For this review, take the finished solid that the model builds, in its own axes (mm). Face numbers are marked on the shaded views. Coordinates: 2 decimals unless noted, no trailing zeros. Loops run counter-clockwise (first coordinate to the right, second up) from the corner with the lowest first, then second, coordinate; pieces in that order, holes last. Notation, with made-up numbers: (86.5, 67.5) -> (112.5, 67.5) arc R10 cw to (112.5, 79.5) -> close; hole circle Ø5 at (1.5, 14). An arc over 180 degrees is marked (long way). One line per item, written item: value.
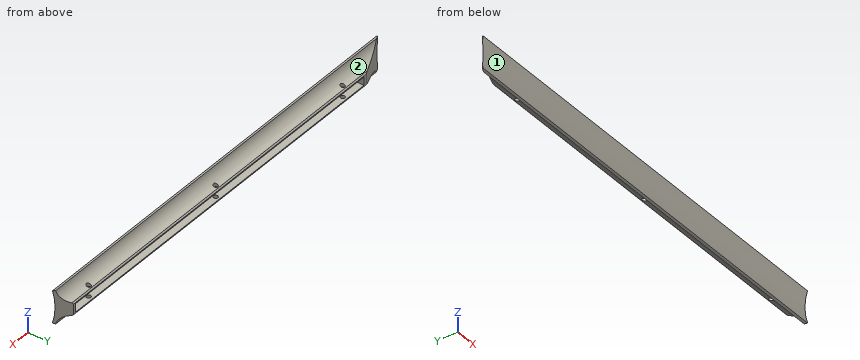
from build123d import *

# Parameters (mm, degrees)
BOSS_EXTRUDE1_DEPTH                 = 254
CUT_EXTRUDE1_DEPTH                  = 263.150751027
SKETCH3_W                           = 425.45
SKETCH3_H                           = 9.525
CUT_EXTRUDE2_DEPTH                  = 9.525
CUT_EXTRUDE3_REACH                  = 257.394
CUT_EXTRUDE3_END_RADIUS             = 15.089603758
SKETCH6_R                           = 2.4384
CUT_EXTRUDE3_DIRECTION_2_REACH      = 257.394
CUT_EXTRUDE3_DIRECTION_2_END_RADIUS = 15.089603758
CHAMFER1_SIZE                       = 1.27


with BuildPart() as part:
    # Sketch1 → Boss-Extrude1 (new, symmetric)
    with BuildSketch(Plane(origin=(0, 0, 0), x_dir=(0, 0, -1), z_dir=(1, 0, 0))):
        with BuildLine():
            Line((-7.1374, 12.7), (7.1374, 12.7))
            ThreePointArc((7.1374, 12.7), (10.363087786, 3.375642683), (18.661047774, -1.962199681))
            Line((18.661047774, -1.962199681), (18.00748716, -4.649455573))
            ThreePointArc((18.00748716, -4.649455573), (0, -2.491135768), (-18.00748716, -4.649455573))
            Line((-18.00748716, -4.649455573), (-18.661047774, -1.962199681))
            ThreePointArc((-18.661047774, -1.962199681), (-10.363087786, 3.375642683), (-7.1374, 12.7))
        make_face()
    extrude(amount=BOSS_EXTRUDE1_DEPTH, both=True)

    # Sketch2 → Cut-Extrude1 (cut, through all)
    with BuildSketch(Plane.XY.offset(44.944976028)):
        Polygon((-254, 12.7), (-215.9, 12.7), (-254, -3.6322), align=None)
        Polygon((254, -4.649455573), (224.3582, -4.649455573), (215.9, 12.7), (254, 12.7), align=None)
    extrude(amount=-CUT_EXTRUDE1_DEPTH, mode=Mode.SUBTRACT)

    # Sketch3 → Cut-Extrude2 (cut)
    with BuildSketch(Plane(origin=(0, 12.7, 0), x_dir=(1, 0, 0), z_dir=(0, 1, 0))):
        Rectangle(SKETCH3_W, SKETCH3_H)
    extrude(amount=-CUT_EXTRUDE2_DEPTH, mode=Mode.SUBTRACT)

    # Cut-Extrude3: up to this cylinder (the profile starts outside it)
    cut_extrude3_end = Plane(origin=(0, 12.7, -22.227003758), z_dir=(-1, 0, 0)) * Cylinder(CUT_EXTRUDE3_END_RADIUS, 920.617207515, mode=Mode.PRIVATE)
    # Sketch6 → Cut-Extrude3 (cut, up to the surface)
    with BuildSketch(Plane.XY.offset(-4.7625), mode=Mode.PRIVATE) as cut_extrude3_sk1:
        with Locations((-187.325, 7.9375)):
            Circle(SKETCH6_R)
    cut_extrude3_tool1 = extrude(cut_extrude3_sk1.sketch, amount=-CUT_EXTRUDE3_REACH, mode=Mode.PRIVATE) - cut_extrude3_end
    add(cut_extrude3_tool1.solids().sort_by_distance((-187.325, 7.9375, -4.7625))[0], mode=Mode.SUBTRACT)
    # Sketch6 → Cut-Extrude3 (cut, up to the surface)
    with BuildSketch(Plane.XY.offset(-4.7625), mode=Mode.PRIVATE) as cut_extrude3_sk2:
        with Locations((187.325, 7.9375)):
            Circle(SKETCH6_R)
    cut_extrude3_tool2 = extrude(cut_extrude3_sk2.sketch, amount=-CUT_EXTRUDE3_REACH, mode=Mode.PRIVATE) - cut_extrude3_end
    add(cut_extrude3_tool2.solids().sort_by_distance((187.325, 7.9375, -4.7625))[0], mode=Mode.SUBTRACT)
    # Sketch6 → Cut-Extrude3 (cut, up to the surface)
    with BuildSketch(Plane.XY.offset(-4.7625), mode=Mode.PRIVATE) as cut_extrude3_sk3:
        with Locations((0, 7.9375)):
            Circle(SKETCH6_R)
    cut_extrude3_tool3 = extrude(cut_extrude3_sk3.sketch, amount=-CUT_EXTRUDE3_REACH, mode=Mode.PRIVATE) - cut_extrude3_end
    add(cut_extrude3_tool3.solids().sort_by_distance((0, 7.9375, -4.7625))[0], mode=Mode.SUBTRACT)

    # Cut-Extrude3 direction 2: up to this cylinder (the profile starts outside it)
    cut_extrude3_direction_2_end = Plane(origin=(0, 12.7, 22.227003758), z_dir=(-1, 0, 0)) * Cylinder(CUT_EXTRUDE3_DIRECTION_2_END_RADIUS, 920.617207515, mode=Mode.PRIVATE)
    # Sketch6 → Cut-Extrude3 direction 2 (cut, up to the surface)
    with BuildSketch(Plane.XY.offset(-4.7625), mode=Mode.PRIVATE) as cut_extrude3_direction_2_sk1:
        with Locations((-187.325, 7.9375)):
            Circle(SKETCH6_R)
    cut_extrude3_direction_2_tool1 = extrude(cut_extrude3_direction_2_sk1.sketch, amount=CUT_EXTRUDE3_DIRECTION_2_REACH, mode=Mode.PRIVATE) - cut_extrude3_direction_2_end
    add(cut_extrude3_direction_2_tool1.solids().sort_by_distance((-187.325, 7.9375, -4.7625))[0], mode=Mode.SUBTRACT)
    # Sketch6 → Cut-Extrude3 direction 2 (cut, up to the surface)
    with BuildSketch(Plane.XY.offset(-4.7625), mode=Mode.PRIVATE) as cut_extrude3_direction_2_sk2:
        with Locations((187.325, 7.9375)):
            Circle(SKETCH6_R)
    cut_extrude3_direction_2_tool2 = extrude(cut_extrude3_direction_2_sk2.sketch, amount=CUT_EXTRUDE3_DIRECTION_2_REACH, mode=Mode.PRIVATE) - cut_extrude3_direction_2_end
    add(cut_extrude3_direction_2_tool2.solids().sort_by_distance((187.325, 7.9375, -4.7625))[0], mode=Mode.SUBTRACT)
    # Sketch6 → Cut-Extrude3 direction 2 (cut, up to the surface)
    with BuildSketch(Plane.XY.offset(-4.7625), mode=Mode.PRIVATE) as cut_extrude3_direction_2_sk3:
        with Locations((0, 7.9375)):
            Circle(SKETCH6_R)
    cut_extrude3_direction_2_tool3 = extrude(cut_extrude3_direction_2_sk3.sketch, amount=CUT_EXTRUDE3_DIRECTION_2_REACH, mode=Mode.PRIVATE) - cut_extrude3_direction_2_end
    add(cut_extrude3_direction_2_tool3.solids().sort_by_distance((0, 7.9375, -4.7625))[0], mode=Mode.SUBTRACT)

    # Chamfer1
    # the kernel refuses this chamfer: 1.27 mm, written as the material it takes off along each edge
    with BuildSketch(Plane(origin=(219.319487902, 12.7, -7.1374), x_dir=(0, 0, 1), z_dir=(-1, 0, 0))) as chamfer1_piece_1:
        with BuildLine():
            Line((CHAMFER1_SIZE, 0), (-0.058604027, -1.328604027))
            ThreePointArc((-0.058604027, -1.328604027), (-0.015497105, -0.683703283), (0, 0))
            Line((0, 0), (CHAMFER1_SIZE, 0))
        make_face()
    extrude(amount=438.638975803, mode=Mode.SUBTRACT)
    with BuildSketch(Plane(origin=(219.319487902, 12.7, 7.1374), x_dir=(0, -0.9990285943565428, 0.04406662748600431), z_dir=(-1, 0, 0))) as chamfer1_piece_2:
        with BuildLine():
            Line((1.329895895, 0), (-CHAMFER1_SIZE * 0.044066627486, -CHAMFER1_SIZE * 0.999028594357))
            Line((-CHAMFER1_SIZE * 0.044066627486, -CHAMFER1_SIZE * 0.999028594357), (0, 0))
            ThreePointArc((0, 0), (0.683722035, -0.014646447), (1.329895895, 0))
        make_face()
    extrude(amount=438.638975803, mode=Mode.SUBTRACT)


solid = part.part
1. Take a section at A-A, the plane x = -68. Give the boundary of the cut face in (y, z) (1 decimal), and give its area (3 significant figures).
Return value:
outline: (-4.6, -18) -> (-2, -18.7) arc R15.1 cw to (11.4, -7.2) -> (12.7, -5.9) -> (12.7, -4.8) -> (3.2, -4.8) -> (3.2, 4.8) -> (12.7, 4.8) -> (12.7, 5.9) -> (11.4, 7.2) arc R15.1 cw to (-2, 18.7) -> (-4.6, 18) arc R76.2 cw to start
area: 250 mm2
2. Insertion check: pin 1 Ø1.5 at (x, y) = (-170.5, 8.5) entering from -Z; pin 2 Ø10 at (x, y) = (-13, 4) entering from +Z; pin 3 Ø5 at (x, y) = (12, 9.5) entering from -Z; pin 4 Ø7.5 at (x, z) = (52.5, 1.5) entering from +Y. Each pin has a flat end and moves straight along its axis. Give the tip position at first contact, or say it passes through.
Return value:
pin 1: stops at z = -7.97
pin 2: stops at z = 15.9
pin 3: stops at z = -8.26
pin 4: stops at y = 12.7
3. To check wall thickness, follow probe 1 along Y at (x, z) = (-122.5, -2) (3 decimals); probe 2 along Z at (x, y) = (84.5, 6.25); probe 3 along X at (y, z) = (10.5, 1) (3 decimals). State the ranges of each line that lie inside material, in increasing order. Write a range as from..to.
Return value:
probe 1: y = -2.517..3.175
probe 2: z = -8.59..-4.76, 4.76..8.59
probe 3: x = -221.032..-212.725, 212.725..216.973
4. The part is to be moulded in two halves that separate along Z. For the marked faces 1 and 2, say which applies: pulls with the +Z half, pulls with the -Z half, needs draft (parallel to the pull), parting line crosses it, or undercut.
Return value:
face 1: undercut
face 2: pulls with the +Z half
